```python
from build123d import *

# Parameters (mm, degrees)
SKETCH_1_R          = 7
EXTRUDE_1_DEPTH     = 28
EXTRUDE_START       = -8
EXTRUDE_2_DEPTH     = 7
SKETCH_6_R          = 5
CUT_EXTRUDE_1_DEPTH = 4
SKETCH_7_R          = 3.175
CUT_EXTRUDE_2_DEPTH = 28.287054318


# Read off the part's stored shape, not the designer's step: M14 机械螺纹 螺柱1, M14 机械螺纹 螺柱2
with BuildPart() as part:
    # 草图1 → 凸台-拉伸1 (new body)
    with BuildSketch(Plane.XY):
        Circle(SKETCH_1_R)
    extrude(amount=EXTRUDE_1_DEPTH)

    # M14 机械螺纹 螺柱1 outline → M14 机械螺纹 螺柱1 (revolve, cut)
    with BuildSketch(Plane.XZ):
        Polygon((7, 28), (5.9175, 28), (7, 26.9175), align=None)
    revolve(axis=Axis((0, 0, 0), (0, 0, 1)), mode=Mode.SUBTRACT)

    # M14 机械螺纹 螺柱2 outline → M14 机械螺纹 螺柱2 (revolve, cut)
    with BuildSketch(Plane.XZ):
        Polygon((7, 1.0825), (5.9175, 0), (7, 0), align=None)
    revolve(axis=Axis((0, 0, 0), (0, 0, 1)), mode=Mode.SUBTRACT)

    # 草图4 → 凸台-拉伸2 (add)
    with BuildSketch(Plane(origin=(0, 0, 0), x_dir=(-1, 0, 0), z_dir=(0, 0, -1)).offset(EXTRUDE_START)):
        Polygon((0, 9.814954576), (-8.5, 4.907477288), (-8.5, -4.907477288), (0, -9.814954576), (8.5, -4.907477288), (8.5, 4.907477288), align=None)
    extrude(amount=-EXTRUDE_2_DEPTH)

    # 草图5 → 切除-旋转1 (revolve, cut)
    with BuildSketch(Plane(origin=(0, 0, 0), x_dir=(0, 0, -1), z_dir=(1, 0, 0)), mode=Mode.PRIVATE) as cut_revolve_1_sk:
        Polygon((-8, 8.50620211), (-8.755608589, 9.814954576), (-8, 9.814954576), align=None)
        Polygon((-15, 8.50620211), (-14.244391411, 9.814954576), (-15, 9.814954576), align=None)
    revolve(cut_revolve_1_sk.sketch.rotate(Axis((0, 0, 0), (0, 0, -1)), 270), axis=Axis((0, 0, 0), (0, 0, -1)), mode=Mode.SUBTRACT)

    # 草图6 → 切除-拉伸1 (cut)
    with BuildSketch(Plane(origin=(0, 0, 0), x_dir=(-1, 0, 0), z_dir=(0, 0, -1))):
        Circle(SKETCH_6_R)
    extrude(amount=-CUT_EXTRUDE_1_DEPTH, mode=Mode.SUBTRACT)

    # 草图7 → 切除-拉伸2 (cut, through all)
    with BuildSketch(Plane(origin=(0, 0, 4), x_dir=(-1, 0, 0), z_dir=(0, 0, -1))):
        Circle(SKETCH_7_R)
    extrude(amount=-CUT_EXTRUDE_2_DEPTH, mode=Mode.SUBTRACT)


solid = part.part
```
Work out the finished part from the listing and answer in its coordinate system (mm). A direction names the side the tool comes from. Give positions to 0.01 mm unless a question says otherwise; leave off trailing zeros. Order: outer loops, then holes, each group sorted by start corner. A loop starts at its lowest first (then second) coordinate and runs counter-clockwise, first axis right, second up.
1. Section B-B, the plane z = 13.5 is taken. Determine the outline of the cut face in (x, y) (3 decimals).
Result sheet:
outline: (-8.5, -4.907) - (0, -9.815) - (8.5, -4.907) - (8.5, 4.907) - (0, 9.815) - (-8.5, 4.907) - close; hole circle Ø6.35 at (0, 0)
2. For faces 1 (the flat face through (-2, -7, 15)), 2 (the cylindrical face through (6.466, -2.681, 4.493)), 3 (the flat face through (4.309, -7.327, 11.451)), determine the directions among +Z, -Z, +X, -X, +Y, -Y from which every point of the face is accessible in a straight line to the end or side of a thin tool.
Result sheet:
face 1: +Z
face 2: -Z
face 3: +Z, -Z, +X, -Y
3. Section A-A, the plane y = 0 is taken. Determine the outline of the cut face in (x, z) (1 decimal).
Result sheet:
outline: (-8.5, 8) - (-7, 8) - (-7, 1.1) - (-5.9, 0) - (-5, 0) - (-5, 4) - (-3.2, 4) - (-3.2, 28) - (-5.9, 28) - (-7, 26.9) - (-7, 15) - (-8.5, 15) - close; (3.2, 4) - (5, 4) - (5, 0) - (5.9, 0) - (7, 1.1) - (7, 8) - (8.5, 8) - (8.5, 15) - (7, 15) - (7, 26.9) - (5.9, 28) - (3.2, 28) - close
4. Straight lines are drawn through the part: L1, parallel to Y at x = 0, z = 1.7; L2, parallel to Y at x = 0, z = 18 (3 decimals); L3, parallel to Z at x = 1.75, y = 3.5. For each, find the intervals that lie inside material, in ascending order.
Result sheet:
L1: y = -7 to -5, 5 to 7
L2: y = -7 to -3.175, 3.175 to 7
L3: z = 4 to 28
5. Each of these flat-tipped pins is pushed along its axis until it touches: P1, Ø1, axis at x = 3.5, y = 4.5, coming from the -Z side; P2, Ø5, axis at x = 5.5, z = 18, coming from the -Y side; P3, Ø3, axis at x = 3, z = 18, coming from the +Y side; P4, Ø8, axis at x = -0.5, y = 0.5, coming from the -Z side. Where does it stop, or does it pass through?
Result sheet:
P1: stops at z = 0
P2: stops at y = -6.32
P3: stops at y = 6.84
P4: stops at z = 4
6. Section C-C, the plane z = 21 is taken. Determine the outline of the cut face in (x, y) (3 decimals), and give its area (3 significant figures).
Result sheet:
outline: circle Ø14 at (0, 0); hole circle Ø6.35 at (0, 0)
area: 122 mm2
